For this review, take the finished solid that the model builds, in its own axes (mm). A direction names the side the tool comes from. Coordinates: 2 decimals unless noted, no trailing zeros. Order: outer loops, then holes, each group sorted by start corner. A loop starts at its lowest first (then second) coordinate and runs counter-clockwise, first axis right, second up.
from build123d import *

# Parameters (mm, degrees)
SKETCH1_W                = 46.5
SKETCH1_H                = 35.6
BOSS_EXTRUDE1_DEPTH      = 2
SKETCH2_W                = 3
SKETCH2_H                = 35.6
BOSS_EXTRUDE2_DEPTH      = 50
SKETCH3_R                = 4.25
CUT_EXTRUDE1_DEPTH       = 47.5
SKETCH6_R                = 1.25
CUT_EXTRUDE3_DEPTH       = 47.5
FILLET5_R                = 16
SKETCH1_2_W              = 46.5
SKETCH1_2_H              = 35.6
CUT_EXTRUDE6_DEPTH       = 20
SKETCH8_W                = 46.5
SKETCH8_H                = 35.6
BOSS_EXTRUDE3_DEPTH      = 3
SKETCH9_W                = 35.6
SKETCH9_H                = 13
BOSS_EXTRUDE4_DEPTH      = 46.5
SKETCH12_W               = 24.4
SKETCH12_H               = 13
CUT_EXTRUDE9_DEPTH       = 36.6
SKETCH13_W               = 30
SKETCH13_H               = 13
CUT_EXTRUDE10_DEPTH      = 36.45
CUT_EXTRUDE10_DEPTH_BACK = 12.05
SKETCH15_R               = 1.35
CUT_EXTRUDE12_DEPTH      = 36.6


with BuildPart() as part:
    # Sketch1 → Boss-Extrude1 (new body)
    with BuildSketch(Plane(origin=(0, 0, 0), x_dir=(1, 0, 0), z_dir=(0, 1, 0))):
        Rectangle(SKETCH1_W, SKETCH1_H)
    extrude(amount=BOSS_EXTRUDE1_DEPTH)

    # Sketch2 → Boss-Extrude2 (add)
    with BuildSketch(Plane(origin=(0, 2, 0), x_dir=(1, 0, 0), z_dir=(0, 1, 0))):
        with Locations((-21.75, 0)):
            Rectangle(SKETCH2_W, SKETCH2_H)
        with Locations((21.75, 0)):
            Rectangle(SKETCH2_W, SKETCH2_H)
    extrude(amount=BOSS_EXTRUDE2_DEPTH)

    # Sketch3 → Cut-Extrude1 (cut, through all)
    with BuildSketch(Plane(origin=(23.25, 0, 0), x_dir=(0, 0, -1), z_dir=(1, 0, 0))):
        with Locations((0, 40)):
            Circle(SKETCH3_R)
    extrude(amount=-CUT_EXTRUDE1_DEPTH, mode=Mode.SUBTRACT)

    # Sketch6 → Cut-Extrude3 (cut, through all)
    with BuildSketch(Plane(origin=(23.25, 0, 0), x_dir=(0, 0, -1), z_dir=(1, 0, 0))):
        with Locations((0, 32)):
            Circle(SKETCH6_R)
        with Locations((-5.656854249, 34.343145751)):
            Circle(SKETCH6_R)
        with Locations((-8, 40)):
            Circle(SKETCH6_R)
        with Locations((-5.656854249, 45.656854249)):
            Circle(SKETCH6_R)
        with Locations((0, 48)):
            Circle(SKETCH6_R)
        with Locations((5.656854249, 45.656854249)):
            Circle(SKETCH6_R)
        with Locations((8, 40)):
            Circle(SKETCH6_R)
        with Locations((5.656854249, 34.343145751)):
            Circle(SKETCH6_R)
    extrude(amount=-CUT_EXTRUDE3_DEPTH, mode=Mode.SUBTRACT)

    # Fillet5
    fillet5_edges = [part.edges().sort_by_distance(p)[0] for p in [
        (-21.75, 52, 17.8),
        (-21.75, 52, -17.8),
        (21.75, 52, -17.8),
        (21.75, 52, 17.8),
    ]]
    fillet(fillet5_edges, radius=FILLET5_R)

    # Sketch1<2> → Cut-Extrude6 (cut)
    with BuildSketch(Plane(origin=(0, 0, 0), x_dir=(1, 0, 0), z_dir=(0, 1, 0))):
        Rectangle(SKETCH1_2_W, SKETCH1_2_H)
    extrude(amount=CUT_EXTRUDE6_DEPTH, mode=Mode.SUBTRACT)

    # Sketch8 → Boss-Extrude3 (add)
    with BuildSketch(Plane.XZ.offset(-20)):
        Rectangle(SKETCH8_W, SKETCH8_H)
    extrude(amount=BOSS_EXTRUDE3_DEPTH)

    # Sketch9 → Boss-Extrude4 (add)
    with BuildSketch(Plane(origin=(23.25, 0, 0), x_dir=(0, 0, -1), z_dir=(1, 0, 0))):
        with Locations((0, 10.5)):
            Rectangle(SKETCH9_W, SKETCH9_H)
    extrude(amount=-BOSS_EXTRUDE4_DEPTH)

    # Sketch12 → Cut-Extrude9 (cut, through all)
    with BuildSketch(Plane(origin=(0, 0, -17.8), x_dir=(-1, 0, 0), z_dir=(0, 0, -1))):
        with Locations((0, 10.5)):
            Rectangle(SKETCH12_W, SKETCH12_H)
    extrude(amount=-CUT_EXTRUDE9_DEPTH, mode=Mode.SUBTRACT)

    # Sketch13 → Cut-Extrude10 (cut, two sides)
    with BuildSketch(Plane.ZY.offset(-12.2)) as cut_extrude10_sk:
        with Locations((0, 10.5)):
            Rectangle(SKETCH13_W, SKETCH13_H)
    extrude(amount=CUT_EXTRUDE10_DEPTH, mode=Mode.SUBTRACT)
    extrude(cut_extrude10_sk.sketch, amount=-CUT_EXTRUDE10_DEPTH_BACK, mode=Mode.SUBTRACT)

    # Sketch15 → Cut-Extrude12 (cut, through all)
    with BuildSketch(Plane(origin=(0, 0, -17.8), x_dir=(-1, 0, 0), z_dir=(0, 0, -1))):
        with Locations((-15, 6.9)):
            Circle(SKETCH15_R)
        with Locations((15, 6.9)):
            Circle(SKETCH15_R)
    extrude(amount=-CUT_EXTRUDE12_DEPTH, mode=Mode.SUBTRACT)


solid = part.part
1. Take a section at C-C, the plane x = -19.5. Give the boundary of the cut face in (y, z), plus the area to 3 significant figures.
Answer below:
outline: (4, -17.8) - (20, -17.8) - (20, 17.8) - (4, 17.8) - (4, 15) - (17, 15) - (17, -15) - (4, -15) - close
area: 180 mm2
2. To check wall thickness, follow L1, parallel to X at y = 30, z = -9; L2, parallel to Z at x = 19.5, y = 13.5. State the ranges of each line that lie inside material, in increasing order.
Answer below:
L1: x = -23.25 to -20.25, 20.25 to 23.25
L2: z = -17.8 to -15, 15 to 17.8
3. Machinability: for faces 4 (the face through (-18, 4, -16)), 5 (the face through (0, 20, 0)), which of the approach directions +Z, -Z, +X, -X, +Y, -Y give a long, thin tool a straight path to every point of the face, cutting with its end or side? Answer none if there is none.
Answer below:
face 4: +Z, -Z, +X, -X, -Y
face 5: +Z, -Z, +Y
4. The part is to be moulded in two halves that separate along Y. For faces 1 (the face through (0, 17, 0)), 2 (the face through (22, 52, 0)), 3 (the face through (21.77, 49.24, 0.16)), say which applies: +Y half, -Y half, draft (parallel to the pull), parting line (faces both ways), or undercut.
Answer below:
face 1: -Y half
face 2: +Y half
face 3: undercut
5. Take a section at D-D, the plane y = 24. Give the boundary of the cut face in (x, z), plus the area to 3 significant figures.
Answer below:
outline: (-23.25, -17.8) - (-20.25, -17.8) - (-20.25, 17.8) - (-23.25, 17.8) - close; (20.25, -17.8) - (23.25, -17.8) - (23.25, 17.8) - (20.25, 17.8) - close
area: 214 mm2
6. Take a section at B-B, the plane y = 6.9. Give the number of separate pieces and of enclosed holes in the cut face, plus the area to 3 significant figures.
Answer below:
separate pieces: 8
enclosed holes: 0
area: 93.5 mm2
7. Take a section at A-A, the plane y = 32. Give the boundary of the cut face in (x, z), plus the area to 3 significant figures.
Answer below:
outline: (-23.25, -17.8) - (-20.25, -17.8) - (-20.25, -1.25) - (-23.25, -1.25) - close; (-23.25, 1.25) - (-20.25, 1.25) - (-20.25, 17.8) - (-23.25, 17.8) - close; (20.25, -17.8) - (23.25, -17.8) - (23.25, -1.25) - (20.25, -1.25) - close; (20.25, 1.25) - (23.25, 1.25) - (23.25, 17.8) - (20.25, 17.8) - close
area: 199 mm2
8. Clearance check with flat-ended pins moving along their axes: pin 1 Ø3 at (y, z) = (48, 0) entering from -X; pin 2 Ø10 at (x, z) = (-13.5, 1) entering from +Y; pin 3 Ø8 at (x, z) = (9, 5.5) entering from -Y. State where each tip first meets the part, or that it passes through.
Answer below:
pin 1: stops at x = -23.25
pin 2: stops at y = 20
pin 3: stops at y = 17
